Can you work these out from the model? Positions are in its coordinate system, mm. A direction names the side the tool comes from. Give positions to 0.01 mm unless a question says otherwise; leave off trailing zeros. Loops run counter-clockwise (first coordinate to the right, second up) from the corner with the lowest first, then second, coordinate; pieces in that order, holes last.
from build123d import *

# Parameters (mm, degrees)
CROQUIS1_W             = 19
CROQUIS1_H             = 10
BRIDA_BASE1_DEPTH      = 2
BRIDA_DE_ARISTA1_DEPTH = 15
CORTAR_EXTRUIR1_REACH  = 62.77
REDONDEO1_R            = 1


# Sheet-metal steps are written as plain solids
with BuildPart() as part:
    # Croquis1 → Brida base1 (new body)
    with BuildSketch(Plane.XY):
        with Locations((9.5, -5)):
            Rectangle(CROQUIS1_W, CROQUIS1_H)
        with BuildLine():
            Line((5.25, -3.5), (5.25, -6.5))
            ThreePointArc((5.25, -6.5), (3.5, -8.25), (1.75, -6.5))
            Line((1.75, -6.5), (1.75, -3.5))
            ThreePointArc((1.75, -3.5), (3.5, -1.75), (5.25, -3.5))
        make_face(mode=Mode.SUBTRACT)
        with BuildLine():
            Line((17.25, -3.5), (17.25, -6.5))
            ThreePointArc((17.25, -6.5), (15.5, -8.25), (13.75, -6.5))
            Line((13.75, -6.5), (13.75, -3.5))
            ThreePointArc((13.75, -3.5), (15.5, -1.75), (17.25, -3.5))
        make_face(mode=Mode.SUBTRACT)
    extrude(amount=-BRIDA_BASE1_DEPTH)

    # Brida de arista1 section (across the edge) → Brida de arista1 (add)
    with BuildSketch(Plane(origin=(17, 2, 0), x_dir=(0, -1, 0), z_dir=(-1, 0, 0))):
        with BuildLine():
            Line((-2, 2), (-2, 56))
            Line((-2, 56), (0, 56))
            Line((0, 56), (0, 2))
            ThreePointArc((0, 2), (0.585786438, 0.585786438), (2, 0))
            Line((2, 0), (2, -2))
            ThreePointArc((2, -2), (-0.828427125, -0.828427125), (-2, 2))
        make_face()
    extrude(amount=BRIDA_DE_ARISTA1_DEPTH)

    # Croquis9 → Cortar-Extruir1 (cut, up to next)
    with BuildSketch(Plane(origin=(0, 4, 0), x_dir=(1, 0, 0), z_dir=(0, 1, 0)), mode=Mode.PRIVATE) as cortar_extruir1_sk1:
        with BuildLine():
            Line((7.75, -11), (7.75, -5))
            ThreePointArc((7.75, -5), (9.5, -3.25), (11.25, -5))
            Line((11.25, -5), (11.25, -11))
            ThreePointArc((11.25, -11), (9.5, -12.75), (7.75, -11))
        make_face()
    cortar_extruir1_tool1 = extrude(cortar_extruir1_sk1.sketch, amount=-CORTAR_EXTRUIR1_REACH, mode=Mode.PRIVATE) & part.part
    # Croquis9 → Cortar-Extruir1 (cut, up to next)
    with BuildSketch(Plane(origin=(0, 4, 0), x_dir=(1, 0, 0), z_dir=(0, 1, 0)), mode=Mode.PRIVATE) as cortar_extruir1_sk2:
        with BuildLine():
            Line((7.75, -51), (7.75, -45))
            ThreePointArc((7.75, -45), (9.5, -43.25), (11.25, -45))
            Line((11.25, -45), (11.25, -51))
            ThreePointArc((11.25, -51), (9.5, -52.75), (7.75, -51))
        make_face()
    cortar_extruir1_tool2 = extrude(cortar_extruir1_sk2.sketch, amount=-CORTAR_EXTRUIR1_REACH, mode=Mode.PRIVATE) & part.part
    add(cortar_extruir1_tool1.solids().sort_by_distance((9.5, 4, 8))[0], mode=Mode.SUBTRACT)
    add(cortar_extruir1_tool2.solids().sort_by_distance((9.5, 4, 48))[0], mode=Mode.SUBTRACT)

    # Redondeo1
    redondeo1_edges = [part.edges().sort_by_distance(p)[0] for p in [
        (17, 3, 56),
        (2, 3, 56),
        (0, 0, -1),
        (19, 0, -1),
        (19, -10, -1),
        (0, -10, -1),
    ]]
    fillet(redondeo1_edges, radius=REDONDEO1_R)


solid = part.part
(1) Thinking about a two-plate mould opening in X: for faces 1 (the flat face through (11.25, 3, 48)), 2 (the flat face through (9, -5, -2)), 3 (the cylindrical face through (16.699, 2.986, 55.715)), which applies, pulls with the +X half, pulls with the -X half, needs draft (parallel to the pull), parting line crosses it, or undercut?
Returned:
face 1: undercut
face 2: needs draft
face 3: pulls with the +X half
(2) Suppose I cut it at C-C on z = 18. List the corners of the cut face in (x, y) for me.
Returned:
outline: (2, 2) - (17, 2) - (17, 4) - (2, 4) - close
(3) Will these pins go through, and if not, where does the flat tip stop? P1, Ø2, axis at y = 2.5, z = 7.5, coming from the -X side; P2, Ø2, axis at y = 3, z = 46.5, coming from the +X side; P3, Ø3, axis at x = 14, y = -3, coming from the +Z side.
Returned:
P1: stops at x = 2
P2: stops at x = 17
P3: stops at z = 0
(4) Please list where these lines run through material, in increasing order: probe 1 along Z at (x, y) = (8.75, 3.25); probe 2 along Y at (x, z) = (6.5, 49); probe 3 along Z at (x, y) = (13.25, -1.75).
Returned:
probe 1: z = -0.33 to 3.42, 12.58 to 43.42, 52.58 to 56
probe 2: y = 2 to 4
probe 3: z = -2 to 0
(5) Suppose I cut it at A-A on x = 8.75. List the corners of the cut face in (y, z) for me.
Returned:
outline: (-10, -2) - (0, -2) arc R4 ccw to (4, 2) - (4, 3.42) - (2, 3.42) - (2, 2) arc R2 cw to (0, 0) - (-10, 0) - close; (2, 12.58) - (4, 12.58) - (4, 43.42) - (2, 43.42) - close; (2, 52.58) - (4, 52.58) - (4, 56) - (2, 56) - close
(6) Which directions (+Z, -Z, +X, -X, +Y, -Y) give clear straight access to the entire face, cutting with the end or side of a thin tool? Please do faces 4 (the cylindrical face through (9.46, 3.01, 43.25)), 5 (the cylindrical face through (15.54, -8.25, -0.99)), 6 (the flat face through (10, 2, 29)), 7 (the flat face through (17.5, 0, -1)).
Returned:
face 4: +Y, -Y
face 5: +Z, -Z
face 6: +Z, +X, -X, -Y
face 7: +Z, -Z, +X, +Y
(7) Suppose I cut it at B-B on x = 12. List the corners of the cut face in (y, z) for me.
Returned:
outline: (-10, -2) - (0, -2) arc R4 ccw to (4, 2) - (4, 56) - (2, 56) - (2, 2) arc R2 cw to (0, 0) - (-10, 0) - close
